Source: CAD feature listing. Evaluate the final solid. Frame: model axes, mm. A direction names the side the tool comes from. Round coordinates to 2 decimals unless told otherwise and drop trailing zeros. Write each loop counter-clockwise with the first axis right and the second up, starting at its lowest first coordinate (ties: lowest second). Pieces come first, ordered by that corner, then holes.
```python
from build123d import *

# Parameters (mm, degrees)
CUT_EXTRUDE2_DEPTH = 6
SKETCH4_OUTSIDE_W  = 18.26
SKETCH4_OUTSIDE_H  = 14.46
CUT_EXTRUDE3_DEPTH = 6.5
FILLET1_R          = 0.5
CUT_EXTRUDE4_START = -1.5
SKETCH5_R          = 3
CUT_EXTRUDE4_DEPTH = 1.5


with BuildPart() as part:
    # Sketch1 → Revolve1 (revolve)
    with BuildSketch(Plane(origin=(0, 0, 0), x_dir=(1, 0, 0), z_dir=(0, 1, 0))):
        with BuildLine():
            ThreePointArc((0, 29), (-4.207271262, 26.701641821), (-4.546615997, 21.919547411))
            Line((-4.546615997, 21.919547411), (-3.1, 18))
            Line((-3.1, 18), (-3.1, 0))
            Line((-3.1, 0), (0, 0))
            Line((0, 0), (0, 29))
        make_face()
    revolve(axis=Axis((0, 0, -29), (0, 0, 1)))

    # Sketch2 → Cut-Extrude2 (cut, symmetric)
    with BuildSketch(Plane(origin=(0, 0, 0), x_dir=(0, 0, -1), z_dir=(1, 0, 0))):
        with BuildLine():
            Line((18, 1.5), (28.769696007, 1.5))
            ThreePointArc((28.769696007, 1.5), (26.031864858, 4.56853644), (21.919547411, 4.546615997))
            Line((21.919547411, 4.546615997), (18, 3.1))
            Line((18, 3.1), (13.400256656, 3.1))
            Line((13.400256656, 3.1), (18, 1.5))
        make_face()
        with BuildLine():
            ThreePointArc((21.919547411, -4.546615997), (26.031864858, -4.56853644), (28.769696007, -1.5))
            Line((28.769696007, -1.5), (18, -1.5))
            Line((18, -1.5), (13.400256656, -3.1))
            Line((13.400256656, -3.1), (18, -3.1))
            Line((18, -3.1), (21.919547411, -4.546615997))
        make_face()
    extrude(amount=CUT_EXTRUDE2_DEPTH, both=True, mode=Mode.SUBTRACT)

    # Sketch4 outside → Cut-Extrude3 (cut)
    with BuildSketch(Plane.XY):
        Rectangle(SKETCH4_OUTSIDE_W, SKETCH4_OUTSIDE_H)
        Polygon((1.55, 2.684678752), (-1.55, 2.684678752), (-3.1, 0), (-1.55, -2.684678752), (1.55, -2.684678752), (3.1, 0), align=None, mode=Mode.SUBTRACT)
    extrude(amount=-CUT_EXTRUDE3_DEPTH, mode=Mode.SUBTRACT)

    # Fillet1
    fillet1_edges = [part.edges().sort_by_distance(p)[0] for p in [
        (2.325, 1.342339376, 0),
        (2.325, -1.342339376, 0),
        (0, -2.684678752, 0),
        (-2.325, -1.342339376, 0),
        (-2.325, 1.342339376, 0),
        (0, 2.684678752, 0),
    ]]
    fillet(fillet1_edges, radius=FILLET1_R)

    # Sketch5 → Cut-Extrude4 (cut, symmetric)
    with BuildSketch(Plane(origin=(0, 1.5, 0), x_dir=(1, 0, 0), z_dir=(0, 1, 0)).offset(CUT_EXTRUDE4_START)):
        with Locations(Location((0, 24, 0), (0, 0, 270))):
            Circle(SKETCH5_R)
    extrude(amount=CUT_EXTRUDE4_DEPTH, both=True, mode=Mode.SUBTRACT)


solid = part.part
```
Q1. Pin query (flat end, axial travel): P1, Ø2.5, axis at x = 0, z = -3, coming from the +Y side; P2, Ø2, axis at x = -3.5, y = -1.5, coming from the -Z side; P3, Ø0.8, axis at x = 2.5, y = -1, coming from the +Z side. Return the tip coordinate at first contact, or that it passes through.
Q2. Section query B-B, the plane x = 0. Output: boundary loops of the cut face in (y, z).
Q3. Section query D-D, the plane z = -18.75. Output: boundary loops of the cut face in (x, y), and give its area (3 significant figures).
Q4. Section query A-A, the plane z = -24. Output: boundary loops of the cut face in (x, y).
Q5. Line query: line 1 (Y direction, x = 2.5, z = -21); line 2 (X direction, y = 0.45, z = -24); line 3 (Y direction, x = 0, z = -2). Output: solid intervals per line, ascending.
Q6. Set-up query: faces 1 (the face through (2.5, -1.4, -6.5)), 2 (the face through (0.404, -3.074, -10.892)), 3 (the face through (0, -2.685, -3)), 4 (the face through (-2.44, 1.45, -6.5)), 5 (the face through (-2.5, -1.4, -6.5)). Return all of +Z, -Z, +X, -X, +Y, -Y with unobstructed straight access to the full face (end or side cutting, diameter ignored); none if empty.
Q7. Section query C-C, the plane z = -15.5. Output: boundary loops of the cut face in (x, y), and give its area (3 significant figures).
Filled in:
1. P1: stops at y = 2.68
1. P2: stops at z = -28.14
1. P3: stops at z = -0.01
2. outline: (-3.1, -13.4) - (-1.5, -18) - (-1.5, -21) - (1.5, -21) - (1.5, -18) - (3.1, -13.4) - (3.1, -6.5) - (2.68, -6.5) - (2.68, -0.5) arc R0.5 ccw to (2.18, 0) - (-2.18, 0) arc R0.5 ccw to (-2.68, -0.5) - (-2.68, -6.5) - (-3.1, -6.5) - close; (-1.5, -28.77) arc R5 ccw to (1.5, -28.77) - (1.5, -27) - (-1.5, -27) - close
3. outline: (-3.03, -1.5) - (3.03, -1.5) arc R3.38 ccw to (3.03, 1.5) - (-3.03, 1.5) arc R3.38 ccw to start
3. area: 19.6 mm2
4. outline: (-4.77, -1.5) - (-3, -1.5) - (-3, 1.5) - (-4.77, 1.5) arc R5 ccw to start; (3, -1.5) - (4.77, -1.5) arc R5 ccw to (4.77, 1.5) - (3, 1.5) - close
5. line 1: y = -1.5 to 1.5
5. line 2: x = -4.98 to -3, 3 to 4.98
5. line 3: y = -2.68 to 2.68
6. face 1: +Z, +X, -Y
6. face 2: +Z
6. face 3: +Z, +X, -X, -Y
6. face 4: +Z, -X, +Y
6. face 5: +Z, -X, -Y
7. outline: (-2, -2.37) - (2, -2.37) arc R3.1 ccw to (2, 2.37) - (-2, 2.37) arc R3.1 ccw to start
7. area: 26.2 mm2
